Design review of the part built by this model. Coordinates are the model's own, in mm. A direction names the side the tool comes from. Coordinates: 2 decimals unless noted, no trailing zeros. Write item = value, one per line. Start each with the question number.
from build123d import *

# Parameters (mm, degrees)
SKETCH1_R           = 1.65
BOSS_EXTRUDE1_DEPTH = 20
BOSS_EXTRUDE2_DEPTH = 3


with BuildPart() as part:
    # Sketch1 → Boss-Extrude1 (new body)
    with BuildSketch(Plane.XY):
        with BuildLine():
            Line((-20, 14), (-20, -14))
            ThreePointArc((-20, -14), (-18.242640687, -18.242640687), (-14, -20))
            Line((-14, -20), (14, -20))
            ThreePointArc((14, -20), (18.242640687, -18.242640687), (20, -14))
            Line((20, -14), (20, 14))
            ThreePointArc((20, 14), (18.242640687, 18.242640687), (14, 20))
            Line((14, 20), (-14, 20))
            ThreePointArc((-14, 20), (-18.242640687, 18.242640687), (-20, 14))
        make_face()
        with Locations((-14, 14)):
            Circle(SKETCH1_R, mode=Mode.SUBTRACT)
        with Locations((-14, -14)):
            Circle(SKETCH1_R, mode=Mode.SUBTRACT)
        with Locations((14, -14)):
            Circle(SKETCH1_R, mode=Mode.SUBTRACT)
        with Locations((14, 14)):
            Circle(SKETCH1_R, mode=Mode.SUBTRACT)
    extrude(amount=BOSS_EXTRUDE1_DEPTH)

    # Sketch3 → Cut-Revolve3 (revolve, cut)
    with BuildSketch(Plane(origin=(0, 0, 0), x_dir=(0, 0, -1), z_dir=(1, 0, 0)), mode=Mode.PRIVATE) as cut_revolve3_sk:
        with BuildLine():
            Line((0, 0), (0, 10))
            Line((0, 10), (-0.79550681, 10))
            ThreePointArc((-0.79550681, 10), (-0.982755606, 10.036386056), (-1.14275142, 10.140248445))
            ThreePointArc((-1.14275142, 10.140248445), (-2.543582926, 11.290569335), (-4.110140926, 12.202415314))
            ThreePointArc((-4.110140926, 12.202415314), (-12.795376332, 11.702503361), (-17, 4.086443629))
            Line((-17, 4.086443629), (-17, 0))
            Line((-17, 0), (0, 0))
        make_face()
        with BuildLine():
            Line((-8, 16.086443629), (-4.110140926, 16.086443629))
            Line((-4.110140926, 16.086443629), (-4.110140926, 25.8))
            Line((-4.110140926, 25.8), (-20, 25.8))
            Line((-20, 25.8), (-20, 4.086443629))
            ThreePointArc((-20, 4.086443629), (-16.485281374, 12.571725004), (-8, 16.086443629))
        make_face()
    revolve(cut_revolve3_sk.sketch.rotate(Axis((0, 0, 22.5), (0, 0, -1)), 90), axis=Axis((0, 0, 22.5), (0, 0, -1)), mode=Mode.SUBTRACT)

    # Sketch4 → Boss-Extrude2 (add)
    # profile 1 of 4: a face of its own
    with BuildSketch(Plane.XY.offset(4.110140926)):
        with BuildLine():
            ThreePointArc((-9.004753668, 14.21797725), (-17.535533906, 17.535533906), (-14.21797725, 9.004753668))
            ThreePointArc((-14.21797725, 9.004753668), (-13.799644035, 8.742473119), (-13.810515536, 8.248838056))
            ThreePointArc((-13.810515536, 8.248838056), (-11.374833375, 11.374833375), (-8.248838056, 13.810515536))
            ThreePointArc((-8.248838056, 13.810515536), (-8.742473119, 13.799644035), (-9.004753668, 14.21797725))
        make_face()
        Polygon((-10.651368439, 14), (-12.325684219, 16.9), (-15.674315781, 16.9), (-17.348631561, 14), (-15.674315781, 11.1), (-12.325684219, 11.1), align=None, mode=Mode.SUBTRACT)
    # profile 2 of 4: a face of its own
    with BuildSketch(Plane.XY.offset(4.110140926)):
        with BuildLine():
            ThreePointArc((14.21797725, 9.004753668), (17.535533906, 17.535533906), (9.004753668, 14.21797725))
            ThreePointArc((9.004753668, 14.21797725), (8.742473119, 13.799644035), (8.248838056, 13.810515536))
            ThreePointArc((8.248838056, 13.810515536), (11.374833375, 11.374833375), (13.810515536, 8.248838056))
            ThreePointArc((13.810515536, 8.248838056), (13.799644035, 8.742473119), (14.21797725, 9.004753668))
        make_face()
        Polygon((17.348631561, 14), (15.674315781, 16.9), (12.325684219, 16.9), (10.651368439, 14), (12.325684219, 11.1), (15.674315781, 11.1), align=None, mode=Mode.SUBTRACT)
    # profile 3 of 4: a face of its own
    with BuildSketch(Plane.XY.offset(4.110140926)):
        with BuildLine():
            ThreePointArc((9.004753668, -14.21797725), (17.535533906, -17.535533906), (14.21797725, -9.004753668))
            ThreePointArc((14.21797725, -9.004753668), (13.799644035, -8.742473119), (13.810515536, -8.248838056))
            ThreePointArc((13.810515536, -8.248838056), (11.374833375, -11.374833375), (8.248838056, -13.810515536))
            ThreePointArc((8.248838056, -13.810515536), (8.742473119, -13.799644035), (9.004753668, -14.21797725))
        make_face()
        Polygon((17.348631561, -14), (15.674315781, -11.1), (12.325684219, -11.1), (10.651368439, -14), (12.325684219, -16.9), (15.674315781, -16.9), align=None, mode=Mode.SUBTRACT)
    # profile 4 of 4: a face of its own
    with BuildSketch(Plane.XY.offset(4.110140926)):
        with BuildLine():
            ThreePointArc((-14.21797725, -9.004753668), (-17.535533906, -17.535533906), (-9.004753668, -14.21797725))
            ThreePointArc((-9.004753668, -14.21797725), (-8.742473119, -13.799644035), (-8.248838056, -13.810515536))
            ThreePointArc((-8.248838056, -13.810515536), (-11.374833375, -11.374833375), (-13.810515536, -8.248838056))
            ThreePointArc((-13.810515536, -8.248838056), (-13.799644035, -8.742473119), (-14.21797725, -9.004753668))
        make_face()
        Polygon((-10.651368439, -14), (-12.325684219, -11.1), (-15.674315781, -11.1), (-17.348631561, -14), (-15.674315781, -16.9), (-12.325684219, -16.9), align=None, mode=Mode.SUBTRACT)
    extrude(amount=BOSS_EXTRUDE2_DEPTH)


solid = part.part
Q1. Clearance check with flat-ended pins moving along their axes: P1, Ø1, axis at x = -10, z = 13.5, coming from the +Y side; P2, Ø4.5, axis at x = -13, y = -13.5, coming from the +Z side; P3, Ø3.5, axis at x = -14.5, z = 6, coming from the -Y side; P4, Ø2, axis at x = -14, y = -14, coming from the +Z side. State where each tip first meets the part, or that it passes through.
Q2. To check wall thickness, follow line 1 (X direction, y = -14, z = 2.4); line 2 (Y direction, x = 0, z = 0.2); line 3 (X direction, y = -14.5, z = 5.5). State the ranges of each line that lie inside material, in increasing order. Write a range as from..to.
Q3. Add section A-A on z = 2. Give the number of separate pieces and of enclosed holes in the cut face, plus the area to 3 significant figures.
Q4. Mouldability with a two-part tool opening along Y and no side actions: class faces 1 (the face through (18.196, -18.289, 2.026)), 2 (the face through (-14.9, -17.1, 7.11)), 3 (the face through (-11.5, 12.53, 5.59)) as released by +Y, released by -Y, zero draft, split by the parting line, or undercut.
Q5. For faces 4 (the face through (-15.4, -15.3, 4.11)), 5 (the face through (-18.196, 18.289, 2.026)), 6 (the face through (-14.9, 17.3, 7.11)), list the 3-axis set-ups (+Z, -Z, +X, -X, +Y, -Y) from which the entire face can be reached by the end or side of a thin tool; tool diameter is ignored.
Values follow:
q1.P1 = 11.4
q1.P2 = 7.11
q1.P3 = -19
q1.P4 = through
q2.line_1 = -20..-15.65, -12.35..12.35, 15.65..20
q2.line_2 = -20..-10, 10..20
q2.line_3 = -18.97..-17.06, -10.94..-9.03, -6.97..6.97, 9.03..10.94, 17.06..18.97
q3.separate_pieces = 1
q3.enclosed_holes = 5
q3.area = 1,160 mm2
q4.face_1 = released by -Y
q4.face_2 = zero draft
q4.face_3 = undercut
q5.face_4 = +Z
q5.face_5 = +Z, -Z, -X, +Y
q5.face_6 = +Z, -X, +Y
